For this review, take the finished solid that the model builds, in its own axes (mm). Coordinates: 2 decimals unless noted, no trailing zeros. Write each loop counter-clockwise with the first axis right and the second up, starting at its lowest first coordinate (ties: lowest second). Pieces come first, ordered by that corner, then holes. Notation, with made-up numbers: (84.5, -15.5) - (126.5, -15.5) arc R26 cw to (126.5, 6.5) - close; hole circle Ø3 at (-29.75, 78.25). An arc over 180 degrees is marked (long way). Use one line per item in the form item = value. Start each with the question number.
1) We need section C-C (x = 16). Give the boundary of the cut face in (y, z).
2) We need section A-A (z = -15.5). Give the boundary of the cut face in (x, y).
3) For L1, parallel to X at y = 4.75, z = 0; L2, parallel to Z at x = -13.5, y = 3; L3, parallel to X at y = 4, z = 90, list the stretches that pass through material, from the lowest coordinate up. Write a range as from..to.
4) Mouldability with a two-part tool opening along X and no side actions: class faces 1 (the cylindrical face through (-36.39, 4.93, -20.22)), 2 (the flat face through (3, 10, 34)), 3 (the cylindrical face through (46.725, 4.93, 47.356)) as pulls with the +X half, pulls with the -X half, needs draft (parallel to the pull), parting line crosses it, or undercut.
5) We need section B-B (x = 0). Give the boundary of the cut face in (y, z), plus the area to 3 significant figures.
6) We need section D-D (z = 0). Give the boundary of the cut face in (x, y), plus the area to 3 significant figures.
7) Insertion check: P1, Ø3, axis at x = -44.5, y = 6, coming from the +Z side; P2, Ø1.5, axis at y = 2.5, z = -21.5, coming from the +X side; P3, Ø6, axis at y = 6.5, z = 12, coming from the -X side; P4, Ø8, axis at x = -23.5, z = 8, coming from the -Y side. Each pin has a flat end and moves straight along its axis. Give the tip position at first contact, or say it passes through.
```python
from build123d import *

# Parameters (mm, degrees)
SKETCH1_R           = 19
SKETCH1_R_2         = 10
BOSS_EXTRUDE1_DEPTH = 10


with BuildPart() as part:
    # Sketch1 → Boss-Extrude1 (new body)
    with BuildSketch(Plane(origin=(0, 0, 0), x_dir=(1, 0, 0), z_dir=(0, 1, 0))):
        with BuildLine():
            ThreePointArc((-41.436781609, 19.680027304), (-64.91984621, 1.788778062), (-45, -20))
            add(Edge.make_bspline(
                [(-45, -20), (-42.951295687, -25.183418909), (-39.715623944, -29.46325745), (-35.29298477, -32.839515621)],
                knots=[0, 0, 0, 0, 0.944416844, 0.944416844, 0.944416844, 0.944416844], degree=3))
            ThreePointArc((-35.29298477, -32.839515621), (-34.497009223, -33.27058744), (-33.607245283, -33.437081025))
            ThreePointArc((-33.607245283, -33.437081025), (-10.495230645, -49.128111854), (-14.943027733, -76.70692202))
            ThreePointArc((-14.943027733, -76.70692202), (-14.395104128, -103.884558947), (12.745045372, -105.413105413))
            ThreePointArc((12.745045372, -105.413105413), (46.894193375, -46.39540437), (34.279777206, 20.61302682))
            ThreePointArc((34.279777206, 20.61302682), (1.604592709, 39.96780307), (-32.517006803, 23.294726197))
            ThreePointArc((-32.517006803, 23.294726197), (-36.453132672, 20.194921951), (-41.436781609, 19.680027304))
        make_face()
        with Locations(Location((0, 0, 0), (0, 0, 270))):
            Circle(SKETCH1_R, mode=Mode.SUBTRACT)
        with Locations(Location((-45, 0, 0), (0, 0, 270))):
            Circle(SKETCH1_R_2, mode=Mode.SUBTRACT)
        with Locations(Location((0, -90, 0), (0, 0, 270))):
            Circle(SKETCH1_R_2, mode=Mode.SUBTRACT)
    extrude(amount=BOSS_EXTRUDE1_DEPTH)


solid = part.part
```
Determined:
q1.outline = (0, -36.66) - (10, -36.66) - (10, -10.25) - (0, -10.25) - close; (0, 10.25) - (10, 10.25) - (10, 102.6) - (0, 102.6) - close
q2.outline = (-57.64, 0) - (-10.99, 0) - (-10.99, 10) - (-57.64, 10) - close; (10.99, 0) - (37.15, 0) - (37.15, 10) - (10.99, 10) - close
q3.L1 = -65..-55, -35..-19, 19..43.63
q3.L2 = -37.65..-13.37, 13.37..43.92, 74.93..104.76
q3.L3 = -20..-10, 10..27.69
q4.face_1 = undercut
q4.face_2 = needs draft
q4.face_3 = pulls with the +X half
q5.outline = (0, -40) - (10, -40) - (10, -19) - (0, -19) - close; (0, 19) - (10, 19) - (10, 80) - (0, 80) - close; (0, 100) - (10, 100) - (10, 110) - (0, 110) - close
q5.area = 920 mm²
q6.outline = (-65, 0) - (-55, 0) - (-55, 10) - (-65, 10) - close; (-35, 0) - (-19, 0) - (-19, 10) - (-35, 10) - close; (19, 0) - (43.63, 0) - (43.63, 10) - (19, 10) - close
q6.area = 506 mm²
q7.P1 = 24.14
q7.P2 = 34.2
q7.P3 = -62.86
q7.P4 = 0
